```python
from build123d import *
from build123d.topology import SkipClean

# Parameters (mm, degrees)
SKETCH_1_R          = 1.985
EXTRUDE_1_DEPTH     = 12
CUT_EXTRUDE_1_DEPTH = 39.218600963
CUT_EXTRUDE_6_DEPTH = 39.218600963
SKETCH_12_R         = 1.985
EXTRUDE_11_DEPTH    = 5
EXTRUDE_START       = 5
SKETCH_13_R         = 1.985
EXTRUDE_12_DEPTH    = 5
SKETCH_14_W         = 2.04
SKETCH_14_H         = 20
CUT_EXTRUDE_7_DEPTH = 41.070705753
SKETCH_15_W         = 6
SKETCH_15_H         = 6
EXTRUDE_13_DEPTH    = 74
SKETCH_17_R         = 2
CUT_EXTRUDE_8_DEPTH = 107.125262104


with BuildPart() as part:
    # 草圖1 → 填料-伸長1 (new body)
    with BuildSketch(Plane.XY):
        with BuildLine():
            Line((-10, 0), (-10, -30.276417548))
            Line((-10, -30.276417548), (10, -30.276417548))
            Line((10, -30.276417548), (10, 0))
            ThreePointArc((10, 0), (0, 10), (-10, 0))
        make_face()
        Circle(SKETCH_1_R, mode=Mode.SUBTRACT)
    extrude(amount=EXTRUDE_1_DEPTH)

    # 草圖2 → 除料-伸長1 (cut, through all)
    with BuildSketch(Plane(origin=(10, 0, 0), x_dir=(0, 0, -1), z_dir=(1, 0, 0))):
        Polygon((-9, 0), (-6, 0), (-3, 0), (-3, 15.780779257), (-9, 15.780779257), align=None)
        Polygon((-3, 0), (-6, 0), (-9, 0), (-8.60053373, -20), (-3, -20), align=None)
    extrude(amount=-CUT_EXTRUDE_1_DEPTH, mode=Mode.SUBTRACT)

    # 草圖11 → 除料-伸長6 (cut, through all)
    with BuildSketch(Plane(origin=(10, 0, 0), x_dir=(0, 0, -1), z_dir=(1, 0, 0))):
        Polygon((-9, 0), (-9, -20), (-8.60053373, -20), align=None)
    extrude(amount=-CUT_EXTRUDE_6_DEPTH, mode=Mode.SUBTRACT)

    # 草圖12 → 填料-伸長11 (add)
    # profile 1 of 2: a face of its own
    with BuildSketch(Plane.XY.offset(12)):
        with BuildLine():
            ThreePointArc((10, 0), (0, 10), (-10, 0))
            ThreePointArc((-10, 0), (0, -10), (10, 0))
        make_face()
        Circle(SKETCH_12_R, mode=Mode.SUBTRACT)
    # profile 2 of 2: a face of its own
    with BuildSketch(Plane.XY.offset(12)):
        with BuildLine():
            ThreePointArc((10, 0), (0, -10), (-10, 0))
            Line((-10, 0), (-10, -30.276417548))
            Line((-10, -30.276417548), (10, -30.276417548))
            Line((10, -30.276417548), (10, 0))
        make_face()
    extrude(amount=EXTRUDE_11_DEPTH)

    # 草圖13 → 填料-伸長12 (add)
    # profile 1 of 2: a face of its own
    with SkipClean():  # the faces are left unmerged after this step: merging them gives an invalid solid
        with BuildSketch(Plane(origin=(0, 0, 0), x_dir=(-1, 0, 0), z_dir=(0, 0, -1)).offset(EXTRUDE_START)):
            with BuildLine():
                ThreePointArc((10, 0), (0, 10), (-10, 0))
                ThreePointArc((-10, 0), (0, -10), (10, 0))
            make_face()
            Circle(SKETCH_13_R, mode=Mode.SUBTRACT)
        # profile 2 of 2: a face of its own
        with BuildSketch(Plane(origin=(0, 0, 0), x_dir=(-1, 0, 0), z_dir=(0, 0, -1)).offset(EXTRUDE_START)):
            with BuildLine():
                ThreePointArc((10, 0), (0, -10), (-10, 0))
                Line((-10, 0), (-10, -30.276417548))
                Line((-10, -30.276417548), (10, -30.276417548))
                Line((10, -30.276417548), (10, 0))
            make_face()
        extrude(amount=-EXTRUDE_12_DEPTH)

    # 草圖14 → 除料-伸長7 (cut, through all)
    with SkipClean():  # the faces are left unmerged after this step: merging them gives an invalid solid
        with BuildSketch(Plane.ZY.offset(10)):
            Polygon((3, 0), (3, -20), (9, -20), (9, 0), (11.04, 0), (11.04, 10), (3, 10), (0.96, 10), (0.96, 0), align=None)
            with Locations((1.98, -10)):
                Rectangle(SKETCH_14_W, SKETCH_14_H)
            with Locations((10.02, -10)):
                Rectangle(SKETCH_14_W, SKETCH_14_H)
        extrude(amount=-CUT_EXTRUDE_7_DEPTH, mode=Mode.SUBTRACT)

    # 草圖15 → 填料-伸長13 (add)
    with SkipClean():  # the faces are left unmerged after this step: merging them gives an invalid solid
        with BuildSketch(Plane.XZ.offset(30.276417548)):
            with Locations((3, 9)):
                Rectangle(SKETCH_15_W, SKETCH_15_H)
            with Locations((-3, 9)):
                Rectangle(SKETCH_15_W, SKETCH_15_H)
            with Locations((3, 3)):
                Rectangle(SKETCH_15_W, SKETCH_15_H)
            with Locations((-3, 3)):
                Rectangle(SKETCH_15_W, SKETCH_15_H)
        extrude(amount=EXTRUDE_13_DEPTH)

    # 草圖17 → 除料-伸長8 (cut, through all)
    with SkipClean():  # the faces are left unmerged after this step: merging them gives an invalid solid
        with BuildSketch(Plane(origin=(0, 0, 0), x_dir=(-1, 0, 0), z_dir=(0, 0, -1))):
            with Locations((0, -100.276417548)):
                Circle(SKETCH_17_R)
        extrude(amount=-CUT_EXTRUDE_8_DEPTH, mode=Mode.SUBTRACT)


solid = part.part
```
Geometry: final body of the model. Coordinates: model frame, mm. A direction names the side the tool comes from. Coordinates: 2 decimals unless noted, no trailing zeros. Order: outer loops, then holes, each group sorted by start corner. A loop starts at its lowest first (then second) coordinate and runs counter-clockwise, first axis right, second up. Notation, with made-up numbers: M 39,58 L 49,58 A15 ccw 49,85 Z; hole C 38.5,74 d6. An arc over 180 degrees is marked long. Answer as CSV lines item,"result".
Q1. First-contact query: P1, Ø3, axis at y = -78.5, z = 8.5, coming from the -X side; P2, Ø1.5, axis at x = 4.5, z = 11, coming from the +Y side; P3, Ø2, axis at x = -4, z = 2, coming from the +Y side. Flat tips, straight axial feed; report the tip coordinate or a pass-through.
Answers:
P1,"stops at x = -6"
P2,"stops at y = 9.27"
P3,"stops at y = -20"
Q2. Draft query along X for faces 4 (the cylindrical face through (0.43, -102.23, 5.92)), 5 (the flat face through (-6, -67, 6)), 6 (the flat face through (0, -67, 0)). Return one class per face: pulls with the +X half, pulls with the -X half, needs draft (parallel to the pull), parting line crosses it, or undercut.
Answers:
face 4,"undercut"
face 5,"pulls with the -X half"
face 6,"needs draft"
Q3. Set-up query: faces 1 (the flat face through (0, -10, -5)), 2 (the flat face through (6, -67, 6)), 3 (the flat face through (0, -67, 12)). Return all of +Z, -Z, +X, -X, +Y, -Y with unobstructed straight access to the full face (end or side cutting, diameter ignored); none if empty.
Answers:
face 1,"-Z, +X, -X, +Y, -Y"
face 2,"+Z, -Z, +X, -Y"
face 3,"+Z, +X, -X, -Y"
Q4. Section A-A on x = 0. Return the cut outline in (y, z) (3 decimals).
Answers:
outline,"M -104.276,0 L -102.276,0 L -102.276,12 L -104.276,12 Z; M -98.276,0 L -30.276,0 L -30.276,-5 L -1.985,-5 L -1.985,0.96 L -20,0.96 L -20,11.04 L -1.985,11.04 L -1.985,17 L -30.276,17 L -30.276,12 L -98.276,12 Z; M 1.985,-5 L 10,-5 L 10,0.96 L 1.985,0.96 Z; M 1.985,11.04 L 10,11.04 L 10,17 L 1.985,17 Z"
Q5. Section B-B on y = -12. Return the cut outline in (x, z), and give its area (3 significant figures).
Answers:
outline,"M -10,-5 L 10,-5 L 10,0.96 L -10,0.96 Z; M -10,11.04 L 10,11.04 L 10,17 L -10,17 Z"
area,"238 mm^2"
Q6. Line query: probe 1 along Y at (x, z) = (0, 0.35) (3 decimals); probe 2 along Y at (x, z) = (0, 6); probe 3 along X at (y, z) = (0, 0.6) (3 decimals). Output: solid intervals per line, ascending. Write a range as [from, to].
Answers:
probe 1,"y = [-104.276, -102.276], [-98.276, -1.985], [1.985, 10]"
probe 2,"y = [-104.28, -102.28], [-98.28, -20]"
probe 3,"x = [-10, -1.985], [1.985, 10]"
Q7. Section C-C on z = -1.75. Return the cut outline in (x, y) (3 decimals).
Answers:
outline,"M -10,-30.276 L 10,-30.276 L 10,0 A10 ccw -10,0 Z; hole C 0,0 d3.97"
Q8. Section D-D on x = -4.5. Return the cut outline in (y, z).
Answers:
outline,"M -104.28,0 L -30.28,0 L -30.28,-5 L 8.93,-5 L 8.93,0.96 L -20,0.96 L -20,11.04 L 8.93,11.04 L 8.93,17 L -30.28,17 L -30.28,12 L -104.28,12 Z"
